Source: CAD feature listing. Evaluate the final solid. Frame: model axes, mm. A direction names the side the tool comes from. Round coordinates to 2 decimals unless told otherwise and drop trailing zeros. Loops run counter-clockwise (first coordinate to the right, second up) from the corner with the lowest first, then second, coordinate; pieces in that order, holes last. Notation, with made-up numbers: (-3, 27) -> (2, 27) arc R13 ccw to (2, 38) -> close; hole circle Ø10 at (-23, -3.75). An arc over 180 degrees is marked (long way). Return JSON: item names as keys, results as strings. Group by question number.
```python
from build123d import *

# Parameters (mm, degrees)
F1_DEPTH = 40
F2_R     = 7.5


with BuildPart() as f1:
    # F0 (on Right) → F1 (new body)
    with BuildSketch(Plane.YZ):
        with BuildLine():
            Line((0, -2), (0, 0))
            ThreePointArc((0, 0), (-19.399179, 5.979998), (-39.598389, 8))
            Line((-39.598389, 8), (-41.598389, 8))
            Line((-41.598389, 8), (-44.510151, 0))
            Line((-44.510151, 0), (-46, 0))
            Line((-46, 0), (-44.180149, 5))
            Line((-44.180149, 5), (-46.180149, 5))
            Line((-46.180149, 5), (-48, 0))
            Line((-48, 0), (-58, 0))
            Line((-58, 0), (-58, 5))
            Line((-58, 5), (-60, 5))
            Line((-60, 5), (-60, -2))
            Line((-60, -2), (0, -2))
        make_face()
    extrude(amount=F1_DEPTH)

    # F2
    f2_edges = [f1.edges().sort_by_distance(p)[0] for p in [
        (20, -48, 0),
    ]]
    fillet(f2_edges, radius=F2_R)


solid = f1.part
```
(1) Set-up query: faces 1 (the face through (20, -56, 0)), 2 (the face through (0, -30, 2)), 3 (the face through (20, -45, 5)). Return all of +Z, -Z, +X, -X, +Y, -Y with unobstructed straight access to the full face (end or side cutting, diameter ignored); none if empty.
(2) Cut plane D-D (y = -8.5). Return loops of the section in (x, z).
(3) Cut plane C-C (z = 1.5). Return loops of the section in (x, y), and give its area (3 significant figures).
(4) Cut plane A-A (z = 4.25). Return loops of the section in (x, y), and give its area (3 significant figures).
(5) Mould query, pull axis Z, two halves, no side actions, for faces 4 (the face through (20, -58, 2)), 5 (the face through (20.28, -48.9, 1.39)), 6 (the face through (19.72, -45.1, 2.47)). Classes: released by +Z, released by -Z, zero draft, split by the parting line, or undercut.
(6) Cut plane B-B (x = 25). Return loops of the section in (y, z).
(7) Pin query (flat end, axial travel): pin 1 (1.5 mm diameter, centred on y = -14.5, z = 3, fed in from -X); pin 2 (2 mm diameter, centred on x = 11.5, y = -59, fed in from +Z); pin 3 (4 mm diameter, centred on x = 14.5, y = -54.5, fed in from +Z); pin 4 (8 mm diameter, centred on x = 31, y = -31.5, fed in from +Z). Return the tip coordinate at first contact, or that it passes through.
(8) Ray query, line 1 (Z direction, x = 15.5, y = -15); line 2 (Z direction, x = 8.5, y = -55). Return the intervals inside material, ascending.
Answers follow:
{
 "1": {"face 1": "+Z, +X, -X", "face 2": "+Z, -Z, -X, +Y, -Y", "face 3": "+Z, +X, -X, -Y"},
 "2": {"outline": "(0, -2) -> (40, -2) -> (40, 3.14) -> (0, 3.14) -> close"},
 "3": {"outline": "(0, -60) -> (40, -60) -> (40, -58) -> (0, -58) -> close; (0, -48.75) -> (40, -48.75) -> (40, -45.45) -> (0, -45.45) -> close; (0, -43.96) -> (40, -43.96) -> (40, -3.77) -> (0, -3.77) -> close", "area": "1,820 mm^2"},
 "4": {"outline": "(0, -60) -> (40, -60) -> (40, -58) -> (0, -58) -> close; (0, -46.49) -> (40, -46.49) -> (40, -44.45) -> (0, -44.45) -> close; (0, -42.96) -> (40, -42.96) -> (40, -12.19) -> (0, -12.19) -> close", "area": "1,390 mm^2"},
 "5": {"face 4": "zero draft", "face 5": "released by +Z", "face 6": "undercut"},
 "6": {"outline": "(-60, -2) -> (0, -2) -> (0, 0) arc R102 ccw to (-39.6, 8) -> (-41.6, 8) -> (-44.51, 0) -> (-46, 0) -> (-44.18, 5) -> (-46.18, 5) -> (-46.2, 4.93) arc R7.5 cw to (-53.25, 0) -> (-58, 0) -> (-58, 5) -> (-60, 5) -> close"},
 "7": {"pin 1": "x = 0", "pin 2": "z = 5", "pin 3": "z = 0.04", "pin 4": "z = 7.92"},
 "8": {"line 1": "-2 to 4.99", "line 2": "-2 to 0"}
}
